Geometry: final body of the model. Coordinates: model frame, mm. Face numbers are marked on the shaded views. A direction names the side the tool comes from. Give positions to 0.01 mm unless a question says otherwise; leave off trailing zeros. Loops run counter-clockwise (first coordinate to the right, second up) from the corner with the lowest first, then second, coordinate; pieces in that order, holes last.
from build123d import *

# Parameters (mm, degrees)
SKETCH_1_R      = 20
EXTRUDE_1_DEPTH = 2
EXTRUDE_2_DEPTH = 20


with BuildPart() as part:
    # 草图1 → 凸台-拉伸1 (new body)
    with BuildSketch(Plane(origin=(0, 0, 0), x_dir=(1, 0, 0), z_dir=(0, 1, 0))):
        with Locations(Location((0, 0, 0), (0, 0, 270))):
            Circle(SKETCH_1_R)
    extrude(amount=EXTRUDE_1_DEPTH)

    # 草图2 → 凸台-拉伸2 (add)
    with BuildSketch(Plane(origin=(0, 2, 0), x_dir=(1, 0, 0), z_dir=(0, 1, 0))):
        Polygon((1.422012769, -15.50129709), (0, -10.377789627), (2.764347063, -9.610554125), (5.438718845, -19.246307109), align=None)
        Polygon((-9.955557418, -11.966587161), (-7.338205419, -7.338205419), (-4.840999439, -8.750376546), (-9.763439294, -17.454949245), align=None)
        Polygon((-15.50129709, -1.422012769), (-10.377789627, 0), (-9.610554125, -2.764347063), (-19.246307109, -5.438718845), align=None)
        Polygon((-11.966587161, 9.955557418), (-7.338205419, 7.338205419), (-8.750376546, 4.840999439), (-17.454949245, 9.763439294), align=None)
        Polygon((-1.422012769, 15.50129709), (0, 10.377789627), (-2.764347063, 9.610554125), (-5.438718845, 19.246307109), align=None)
        Polygon((9.955557418, 11.966587161), (7.338205419, 7.338205419), (4.840999439, 8.750376546), (9.763439294, 17.454949245), align=None)
        Polygon((15.50129709, 1.422012769), (10.377789627, 0), (9.610554125, 2.764347063), (19.246307109, 5.438718845), align=None)
        Polygon((11.966587161, -9.955557418), (7.338205419, -7.338205419), (8.750376546, -4.840999439), (17.454949245, -9.763439294), align=None)
    extrude(amount=EXTRUDE_2_DEPTH)


solid = part.part
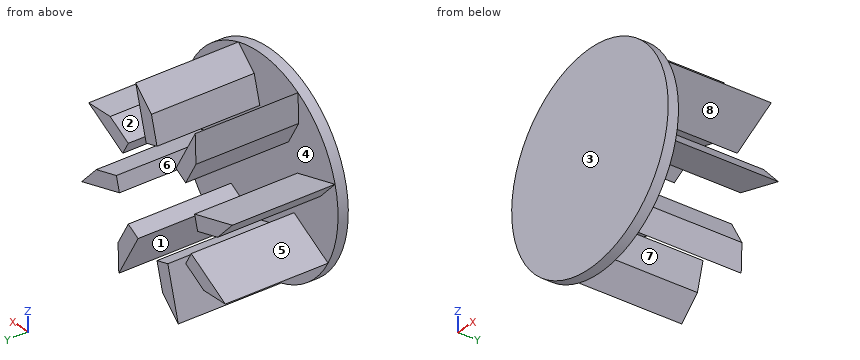
Item 1: Draft query along X for the marked faces 6, 7 and 8. Return one class per face: +X half, -X half, draft (parallel to the pull), parting line (faces both ways), or undercut.
Values follow:
face 6: -X half
face 7: undercut
face 8: +X half
Item 2: Section query A-A on y = 8.75. Give the number of separate pieces and of enclosed holes in the cut face, plus the area to 3 significant figures.
Values follow:
separate pieces: 8
enclosed holes: 0
area: 176 mm2
Item 3: Set-up query: the marked faces 1, 2, 3, 4 and 5. Return all of +Z, -Z, +X, -X, +Y, -Y with unobstructed straight access to the full face (end or side cutting, diameter ignored); none if empty.
Values follow:
face 1: -Z, +Y
face 2: +Z, +Y
face 3: +Z, -Z, +X, -X, -Y
face 4: +Y
face 5: -X, +Y
Item 4: Section query B-B on z = 3.5. Return loops of the section in (x, y), plus the area to 3 significant figures.
Values follow:
outline: (-19.69, 0) - (19.69, 0) - (19.69, 2) - (-12.26, 2) - (-12.26, 22) - (-17.44, 22) - (-17.44, 2) - (-19.69, 2) - close
area: 182 mm2
Item 5: Ray query, probe 1 along Y at (x, z) = (5.5, -7.5); probe 2 along Z at (x, y) = (-12.5, 17); probe 3 along Z at (x, y) = (15.5, 4). Return the intervals inside material, ascending.
Values follow:
probe 1: y = 0 to 2
probe 2: z = -9.94 to -6.96, 0.59 to 3.57
probe 3: z = -4.4 to -1.42, 8.66 to 9.83
Item 6: Section query C-C on x = -8. Return loops of the section in (y, z), plus the area to 3 significant figures.
Values follow:
outline: (0, -18.33) - (2, -18.33) - (2, -7.71) - (22, -7.71) - (22, -6.17) - (2, -6.17) - (2, 8.51) - (22, 8.51) - (22, 14.34) - (2, 14.34) - (2, 18.33) - (0, 18.33) - close
area: 221 mm2
Item 7: Section query D-D on x = -15. Return loops of the section in (y, z), plus the area to 3 significant figures.
Values follow:
outline: (0, -13.23) - (2, -13.23) - (2, -9.85) - (22, -9.85) - (22, -8.38) - (2, -8.38) - (2, 1.28) - (22, 1.28) - (22, 4.26) - (2, 4.26) - (2, 13.23) - (0, 13.23) - close
area: 142 mm2
Item 8: Pin query (flat end, axial travel): pin 1 (5 mm diameter, centred on y = 18, z = 5, fed in from -X); pin 2 (1.5 mm diameter, centred on y = 4, z = 9.5, fed in from +X); pin 3 (1 mm diameter, centred on x = -0.5, z = 13, fed in from +Y). Return the tip coordinate at first contact, or that it passes through.
Values follow:
pin 1: stops at x = -19.25
pin 2: stops at x = 17.45
pin 3: stops at y = 2
